Source: CAD feature listing. Evaluate the final solid. Frame: model axes, mm. A direction names the side the tool comes from. Coordinates: 2 decimals unless noted, no trailing zeros. Write each loop counter-clockwise with the first axis right and the second up, starting at its lowest first coordinate (ties: lowest second). Pieces come first, ordered by that corner, then holes. Notation, with made-up numbers: (31.25, -30) - (75.25, -30) arc R10 ccw to (75.25, -23) - close; hole circle Ø4 at (54.5, 36). An arc over 180 degrees is marked (long way). One line per item, written item: value.
Autodesk Inventor part; units mm, degrees
ref_plane "YZ Plane" through (0, 0, 0) normal (1, 0, 0) x (0, 1, 0)
ref_plane "XZ Plane" through (0, 0, 0) normal (0, 1, 0) x (-1, 0, 0)
ref_plane "XY Plane" through (0, 0, 0) normal (0, 0, 1) x (1, 0, 0)
sketch "Sketch1" plane through (0, 0, 0) normal (1, 0, 0) x (0, 1, 0)
  line L0 (0, 0) -> (0, -28) construction
  line L1 (0, 0) -> (2, 0)
  line L2 (2, 0) -> (2, -5)
  line L3 (2, -5) -> (0, -5)
  line L4 (0, -5) -> (0, 0)
  line L5 (0, -5) -> (1.5, -5)
  line L6 (1.5, -5) -> (1.5, -14)
  line L7 (1.5, -14) -> (0, -14)
  line L8 (0, -14) -> (0, -5)
  line L9 (0, -14) -> (1.25, -14)
  line L10 (1.25, -14) -> (1.25, -28)
  line L11 (1.25, -28) -> (0, -28)
  line L12 (0, -28) -> (0, -14)
  line L13 (1.5, -4) -> (1.5, 0)
  line L14 (0, -4) -> (1.5, -4)
  line L15 (2, 0) -> (1.5, 0)
  line L16 (0, -4) -> (0, -5)
  dimension "d0" = 28
  dimension "d2" = 5
  dimension "d5" = 9
  dimension "d6" = 3
  dimension "d7" = 1.25
  dimension "d23" = 4
  dimension "d24" = 0.5
revolve "Revolution1" add sketch "Sketch1" angle 360 about axis through (0, 0, 0) along (0, 0, -1) contours L1 L2 L3 L4 L14 L13 | L3 L6 L7 L8 | L7 L10 L11 L12
sketch "Sketch2" plane through (0, 0, 0) normal (0, 0, 1) x (1, 0, 0)
  line L0 (0, 0) -> (0, 5.9662) construction
  circle A0 centre (0, 0) radius 2
  line L1 (0, 0) -> (0, -6.6565) construction
  line L2 (0, 0) -> (4.6514, 0) construction
  line L3 (0, 0) -> (-5.9334, 0) construction
  line L4 (1.9984, -0.08) -> (1.4967, -0.1)
  line L5 (0.1, -1.9975) -> (0.1, -1.4967)
  line L6 (1.4967, -0.1) -> (1.9984, -0.08)
  circle A1 centre (0, 0) radius 1.5
  line L7 (0.1, 1.4967) -> (0.1, 1.9975)
  line L8 (-0.1, 1.4967) -> (-0.1, 1.9975)
  line L9 (-1.4967, 0.1) -> (-1.9984, 0.08)
  line L10 (-1.4967, -0.1) -> (-1.9984, -0.08)
  line L11 (-0.08, -1.9984) -> (-0.1, -1.4967)
  line L12 (1.4967, 0.1) -> (1.9984, 0.08)
  line L13 (1.9984, 0.08) -> (1.4967, 0.1)
  dimension "d14" = 0.1
extrude "Extrusion1" cut sketch "Sketch2" against normal blind 0.5 contours A0 L4 A1 L12 | L7 A1 L8 A0 | A0 L11 A1 L5 | L9 A1 L10 A0
chamfer "Chamfer1" distance 0.3 angle 45 4 edges at (1.0607, 1.0607, 0) (-1.0607, 1.0607, 0) (-1.0607, -1.0607, 0) (1.0607, -1.0607, 0)
thread "Thread1"
properties part number "PINO DO BLOCO DE CONTATO" material "Aluminum 6061-AHC"
1) Reachability of faces 4 (the cylindrical face through (-0.766, 1.847, -2.535)), 5 (the conical face through (-1.14, 1.15, -0.18)), 6 (the cylindrical face through (-1.22, -0.27, -21.1)) from +Z, -Z, +X, -X, +Y, -Y: full face, straight path, thin tool, end or side. Return the list, or none.
Values found:
face 4: +Z, -Z
face 5: +Z
face 6: -Z
2) Draft query along Y for faces 1 (the cylindrical face through (0.07, -1.5, -9.56)), 2 (the flat face through (0, 0, -28)), 3 (the conical face through (1.16, 1.13, -0.18)). Return one class per face: released by +Y, released by -Y, zero draft, split by the parting line, or undercut.
Values found:
face 1: split by the parting line
face 2: zero draft
face 3: undercut
3) Section query A-A on z = -3.25. Output: boundary loops of the cut face in (x, y), then the cut area to 3 significant figures.
Values found:
outline: circle Ø4 at (0, 0); hole circle Ø3 at (0, 0)
area: 5.50 mm2
4) Section query B-B on z = -23.25. Output: boundary loops of the cut face in (x, y).
Values found:
outline: circle Ø2.5 at (0, 0)
5) Material intervals for line 1 (X direction, y = 0, z = -2.5); line 2 (Z direction, x = 1.1, y = 1.6), sorted ascending.
Values found:
line 1: -2 to -1.5, 1.5 to 2
line 2: -5 to 0
6) Contact query for flat-ended pins moving along their axis: P1, Ø2, axis at y = 0.5, z = -14, coming from the -X side; P2, Ø1.8, axis at x = 0, y = 0, coming from the +Z side. Output: stop coordinate, or through.
Values found:
P1: x = -1.5
P2: z = -4
